Input: part model. Units: mm. Frame: model coordinates. A direction names the side the tool comes from. Coordinates: 2 decimals unless noted, no trailing zeros. Order: outer loops, then holes, each group sorted by start corner. A loop starts at its lowest first (then second) coordinate and runs counter-clockwise, first axis right, second up. Notation, with made-up numbers: (61, 58) -> (102, 58) arc R5 cw to (102, 64) -> close; hole circle Ø3 at (6, 7.25). An arc over 180 degrees is marked (long way). One line per question, with ' | ' between items.
```python
from build123d import *

# Parameters (mm, degrees)
BOSS_EXTRUDE18_DEPTH            = 24.1
CUT_EXTRUDE24_DEPTH             = 10.3
CUT_EXTRUDE25_DEPTH             = 8.9
BOSS_EXTRUDE7_DEPTH             = 9.3
CUT_EXTRUDE21_START             = -2
CUT_EXTRUDE21_DEPTH             = 2
BOSS_EXTRUDE2_REACH             = 48.304
SKETCH16_W                      = 40.7
SKETCH16_H                      = 7
BOSS_EXTRUDE2_DIRECTION_2_REACH = 48.304
BOSS_EXTRUDE3_REACH             = 58.743
SKETCH23_R                      = 3.5
BOSS_EXTRUDE3_DIRECTION_2_REACH = 58.743
SKETCH24_W                      = 12
SKETCH24_H                      = 5.4
SKETCH24_H_2                    = 3.45
CUT_EXTRUDE6_DEPTH              = 66.882774684
BOSS_EXTRUDE4_DEPTH             = 1
BOSS_EXTRUDE4_DEPTH_BACK        = 2.6
SKETCH28_R                      = 3
SKETCH33_W                      = 2.6
SKETCH33_H                      = 4
CUT_EXTRUDE10_DEPTH             = 5.4
CUT_EXTRUDE12_DEPTH             = 2.5
DELETEFACE7_START               = 23.1
DELETEFACE7_DEPTH               = 1
CUT_EXTRUDE29_START             = -1
SKETCH105_R                     = 1.7
CUT_EXTRUDE29_DEPTH             = 1
SKETCH106_W                     = 18
SKETCH106_H                     = 31.4
CUT_EXTRUDE30_DEPTH             = 2
CUT_EXTRUDE31_DEPTH             = 1.4


# Read off the part's stored shape, not the designer's step: DeleteFace7
with BuildPart() as part:
    # Sketch95 → Boss-Extrude18 (new body)
    with BuildSketch(Plane(origin=(0, 0, 0), x_dir=(0, 0, -1), z_dir=(1, 0, 0))):
        with BuildLine():
            Line((9, 29.5), (9, 7.1))
            Line((9, 7.1), (8.45, 7.1))
            Line((8.45, 7.1), (8.45, 0))
            Line((8.45, 0), (-8.45, 0))
            Line((-8.45, 0), (-8.45, 7.1))
            Line((-8.45, 7.1), (-9, 7.1))
            Line((-9, 7.1), (-9, 29.5))
            ThreePointArc((-9, 29.5), (0, 38.5), (9, 29.5))
        make_face()
    extrude(amount=BOSS_EXTRUDE18_DEPTH)

    # Sketch96 → Cut-Extrude24 (cut)
    with BuildSketch(Plane(origin=(24.1, 0, 0), x_dir=(0, 0, -1), z_dir=(1, 0, 0))):
        with BuildLine():
            Line((-7.45, 8.1), (-7.45, 1))
            Line((-7.45, 1), (7.45, 1))
            Line((7.45, 1), (7.45, 8.1))
            Line((7.45, 8.1), (8, 8.1))
            Line((8, 8.1), (8, 21.5))
            ThreePointArc((8, 21.5), (6.894427191, 23.288854382), (4.8, 23.1))
            ThreePointArc((4.8, 23.1), (0, 21.5), (-4.8, 23.1))
            ThreePointArc((-4.8, 23.1), (-6.894427191, 23.288854382), (-8, 21.5))
            Line((-8, 21.5), (-8, 8.1))
            Line((-8, 8.1), (-7.45, 8.1))
        make_face()
    extrude(amount=-CUT_EXTRUDE24_DEPTH, mode=Mode.SUBTRACT)

    # Sketch97 → Cut-Extrude25 (cut)
    with BuildSketch(Plane(origin=(24.1, 0, 0), x_dir=(0, 0, -1), z_dir=(1, 0, 0))):
        with BuildLine():
            Line((-8, 29.5), (-8, 21.5))
            Line((-8, 21.5), (8, 21.5))
            Line((8, 21.5), (8, 29.5))
            ThreePointArc((8, 29.5), (0, 37.5), (-8, 29.5))
        make_face()
    extrude(amount=-CUT_EXTRUDE25_DEPTH, mode=Mode.SUBTRACT)

    # Sketch11 → Cut-Revolve1 (revolve, cut)
    with BuildSketch(Plane.XY):
        Polygon((13.8, 14.5), (13.8, 9), (1.5, 9), (1.5, 10.25), (0, 10.25), (0, 14.5), align=None)
    revolve(axis=Axis((19.869277651, 14.5, 0), (-1, 0, 0)), mode=Mode.SUBTRACT)

    # Sketch12 → Cut-Revolve2 (revolve, cut)
    with BuildSketch(Plane.XY, mode=Mode.PRIVATE) as cut_revolve2_sk:
        Polygon((15.2, 29.5), (15.2, 26), (13.6, 26), (13.6, 22.25), (0, 22.25), (0, 29.5), align=None)
    revolve(cut_revolve2_sk.sketch.rotate(Axis((8.225974271, 29.5, 0), (1, 0, 0)), 270), axis=Axis((8.225974271, 29.5, 0), (1, 0, 0)), mode=Mode.SUBTRACT)

    # Sketch69 → Boss-Extrude7 (add)
    with BuildSketch(Plane(origin=(13.8, 0, 0), x_dir=(0, 0, -1), z_dir=(1, 0, 0))):
        with BuildLine():
            Line((8, 23.75), (8, 20.25))
            Line((8, 20.25), (6.25, 20.25))
            ThreePointArc((6.25, 20.25), (4.5, 22), (6.25, 23.75))
            Line((6.25, 23.75), (8, 23.75))
        make_face()
        with BuildLine():
            Line((-8, 23.75), (-8, 20.25))
            Line((-8, 20.25), (-6.25, 20.25))
            ThreePointArc((-6.25, 20.25), (-4.5, 22), (-6.25, 23.75))
            Line((-6.25, 23.75), (-8, 23.75))
        make_face()
        with BuildLine():
            Line((-4.6, 2.4), (-4.6, 1))
            Line((-4.6, 1), (-1.2, 1))
            Line((-1.2, 1), (-1.2, 2.4))
            ThreePointArc((-1.2, 2.4), (-2.9, 4.1), (-4.6, 2.4))
        make_face()
    extrude(amount=BOSS_EXTRUDE7_DEPTH)

    # Sketch80 → Cut-Extrude21 (cut)
    with BuildSketch(Plane(origin=(24.1, 0, 0), x_dir=(0, 0, -1), z_dir=(1, 0, 0)).offset(CUT_EXTRUDE21_START)):
        with BuildLine():
            Line((-7.45, 0), (-9, 0))
            Line((-9, 0), (-9, 8.1))
            Line((-9, 8.1), (-7.45, 8.1))
            Line((-7.45, 8.1), (-7.45, 2.4))
            Line((-7.45, 2.4), (-4.6, 2.4))
            ThreePointArc((-4.6, 2.4), (-2.9, 0.7), (-1.2, 2.4))
            Line((-1.2, 2.4), (7.45, 2.4))
            Line((7.45, 2.4), (7.45, 8.1))
            Line((7.45, 8.1), (9, 8.1))
            Line((9, 8.1), (9, 0))
            Line((9, 0), (7.45, 0))
            Line((7.45, 0), (-7.45, 0))
        make_face()
    extrude(amount=CUT_EXTRUDE21_DEPTH, mode=Mode.SUBTRACT)

    # Boss-Extrude2: up to this face of the body (flat: up to its plane)
    boss_extrude2_end = Plane(part.part.faces().sort_by_distance((11.05, 3.55, 8.45))[0])
    # Sketch16 → Boss-Extrude2 (add, up to the picked face)
    with BuildSketch(Plane.XY, mode=Mode.PRIVATE) as boss_extrude2_sk1:
        with Locations((-20.35, 3.5)):
            Rectangle(SKETCH16_W, SKETCH16_H)
    boss_extrude2_tool1 = split(extrude(boss_extrude2_sk1.sketch, amount=BOSS_EXTRUDE2_REACH, mode=Mode.PRIVATE), bisect_by=boss_extrude2_end, keep=Keep.BOTH, mode=Mode.PRIVATE)
    add(boss_extrude2_tool1.solids().sort_by(Axis((-20.35, 3.5, 0), (0, 0, 1)))[0])

    # Boss-Extrude2 direction 2: up to this face of the body (flat: up to its plane)
    boss_extrude2_direction_2_end = Plane(part.part.faces().sort_by_distance((11.05, 3.55, -8.45))[0])
    # Sketch16 → Boss-Extrude2 direction 2 (add, up to the picked face)
    with BuildSketch(Plane.XY, mode=Mode.PRIVATE) as boss_extrude2_direction_2_sk1:
        with Locations((-20.35, 3.5)):
            Rectangle(SKETCH16_W, SKETCH16_H)
    boss_extrude2_direction_2_tool1 = split(extrude(boss_extrude2_direction_2_sk1.sketch, amount=-BOSS_EXTRUDE2_DIRECTION_2_REACH, mode=Mode.PRIVATE), bisect_by=boss_extrude2_direction_2_end, keep=Keep.BOTH, mode=Mode.PRIVATE)
    add(boss_extrude2_direction_2_tool1.solids().sort_by(Axis((-20.35, 3.5, 0), (0, 0, -1)))[0])

    # Boss-Extrude3: up to this face of the body (flat: up to its plane)
    boss_extrude3_end = Plane(part.part.faces().sort_by_distance((-9.198206243, 3.517757633, 8.45))[0])
    # Sketch23 → Boss-Extrude3 (add, up to the picked face)
    with BuildSketch(Plane.XY, mode=Mode.PRIVATE) as boss_extrude3_sk1:
        with BuildLine():
            Line((-41.908497378, 7), (-40.7, 7))
            Line((-40.7, 7), (-40.7, 0))
            Line((-40.7, 0), (-47.2, 0))
            ThreePointArc((-47.2, 0), (-51.587482194, 8.81662479), (-41.908497378, 7))
        make_face()
        with Locations(Location((-47.2, 5.5, 0), (0, 0, 180))):
            Circle(SKETCH23_R, mode=Mode.SUBTRACT)
    boss_extrude3_tool1 = split(extrude(boss_extrude3_sk1.sketch, amount=BOSS_EXTRUDE3_REACH, mode=Mode.PRIVATE), bisect_by=boss_extrude3_end, keep=Keep.BOTH, mode=Mode.PRIVATE)
    add(boss_extrude3_tool1.solids().sort_by(Axis((-41.304249, 6.837212, 0), (0, 0, 1)))[0])

    # Boss-Extrude3 direction 2: up to this face of the body (flat: up to its plane)
    boss_extrude3_direction_2_end = Plane(part.part.faces().sort_by_distance((-9.198206243, 3.517757633, -8.45))[0])
    # Sketch23 → Boss-Extrude3 direction 2 (add, up to the picked face)
    with BuildSketch(Plane.XY, mode=Mode.PRIVATE) as boss_extrude3_direction_2_sk1:
        with BuildLine():
            Line((-41.908497378, 7), (-40.7, 7))
            Line((-40.7, 7), (-40.7, 0))
            Line((-40.7, 0), (-47.2, 0))
            ThreePointArc((-47.2, 0), (-51.587482194, 8.81662479), (-41.908497378, 7))
        make_face()
        with Locations(Location((-47.2, 5.5, 0), (0, 0, 180))):
            Circle(SKETCH23_R, mode=Mode.SUBTRACT)
    boss_extrude3_direction_2_tool1 = split(extrude(boss_extrude3_direction_2_sk1.sketch, amount=-BOSS_EXTRUDE3_DIRECTION_2_REACH, mode=Mode.PRIVATE), bisect_by=boss_extrude3_direction_2_end, keep=Keep.BOTH, mode=Mode.PRIVATE)
    add(boss_extrude3_direction_2_tool1.solids().sort_by(Axis((-41.304249, 6.837212, 0), (0, 0, -1)))[0])

    # Sketch24 → Cut-Extrude6 (cut, through all)
    with BuildSketch(Plane(origin=(0, 0, 0), x_dir=(1, 0, 0), z_dir=(0, 1, 0))):
        with Locations((-46.7, 0)):
            Rectangle(SKETCH24_W, SKETCH24_H)
        with Locations((-46.7, -6.725)):
            Rectangle(SKETCH24_W, SKETCH24_H_2)
        with Locations((-46.7, 6.725)):
            Rectangle(SKETCH24_W, SKETCH24_H_2)
    extrude(amount=CUT_EXTRUDE6_DEPTH, mode=Mode.SUBTRACT)

    # Sketch28 → Boss-Extrude4 (add, two sides: drawn at the far end of the back side and taken through both)
    with BuildSketch(Plane(origin=(-40.7, 0, 0), x_dir=(0, 0, -1), z_dir=(1, 0, 0)).offset(-BOSS_EXTRUDE4_DEPTH_BACK)):
        with BuildLine():
            Line((-5, 7), (5, 7))
            Line((5, 7), (5, 14.5))
            ThreePointArc((5, 14.5), (0, 19.5), (-5, 14.5))
            Line((-5, 14.5), (-5, 7))
        make_face()
        with Locations((0, 14.5)):
            Circle(SKETCH28_R, mode=Mode.SUBTRACT)
    extrude(amount=BOSS_EXTRUDE4_DEPTH + BOSS_EXTRUDE4_DEPTH_BACK)

    # Sketch33 → Cut-Extrude10 (cut)
    with BuildSketch(Plane.XY.offset(-2.7)):
        with Locations((-42, 7)):
            Rectangle(SKETCH33_W, SKETCH33_H)
    extrude(amount=CUT_EXTRUDE10_DEPTH, mode=Mode.SUBTRACT)

    # Sketch35 → Cut-Extrude12 (cut)
    with BuildSketch(Plane(origin=(0, 7, 0), x_dir=(1, 0, 0), z_dir=(0, 1, 0))):
        Polygon((-36.6, 2.65), (-38.1, 2.65), (-38.1, -2.65), (-36.6, -2.65), (-8.3, -2.65), (-6.8, -2.65), (-6.8, 2.65), (-8.3, 2.65), align=None)
    extrude(amount=-CUT_EXTRUDE12_DEPTH, mode=Mode.SUBTRACT)

    # DeleteFace7 outline → DeleteFace7 (cut)
    with BuildSketch(Plane.YZ.offset(DELETEFACE7_START)):
        with BuildLine():
            Line((1, 1.935634924), (1, 3.864365076))
            ThreePointArc((1, 3.864365076), (0.7, 2.9), (1, 1.935634924))
        make_face()
    extrude(amount=DELETEFACE7_DEPTH, mode=Mode.SUBTRACT)

    # Sketch105 → Cut-Extrude29 (cut)
    with BuildSketch(Plane(origin=(23.1, 0, 0), x_dir=(0, 0, -1), z_dir=(1, 0, 0)).offset(CUT_EXTRUDE29_START)):
        with Locations((-2.9, 2.4)):
            Circle(SKETCH105_R)
    extrude(amount=CUT_EXTRUDE29_DEPTH, mode=Mode.SUBTRACT)

    # Sketch106 → Cut-Extrude30 (cut)
    with BuildSketch(Plane(origin=(24.1, 0, 0), x_dir=(0, 0, -1), z_dir=(1, 0, 0))):
        with Locations((0, 22.8)):
            Rectangle(SKETCH106_W, SKETCH106_H)
    extrude(amount=-CUT_EXTRUDE30_DEPTH, mode=Mode.SUBTRACT)

    # Sketch107 → Cut-Extrude31 (cut)
    with BuildSketch(Plane(origin=(15.2, 0, 0), x_dir=(0, 0, -1), z_dir=(1, 0, 0))):
        with BuildLine():
            Line((-6.25, 23.75), (6.25, 23.75))
            ThreePointArc((6.25, 23.75), (5.583042256, 23.617920693), (5.016760303, 23.241619849))
            ThreePointArc((5.016760303, 23.241619849), (4.906085954, 23.174321373), (4.8, 23.1))
            ThreePointArc((4.8, 23.1), (0, 21.5), (-4.8, 23.1))
            ThreePointArc((-4.8, 23.1), (-4.906085954, 23.174321373), (-5.016760303, 23.241619849))
            ThreePointArc((-5.016760303, 23.241619849), (-5.583042256, 23.617920693), (-6.25, 23.75))
        make_face()
    extrude(amount=-CUT_EXTRUDE31_DEPTH, mode=Mode.SUBTRACT)


solid = part.part
```
1. Mould query, pull axis Z, two halves, no side actions, for faces 4 (the face through (18, 14, 8)), 5 (the face through (-50.433, 6.841, -3.834)), 6 (the face through (-10, 4, 8.45)). Classes: released by +Z, released by -Z, zero draft, split by the parting line, or undercut.
Recorded:
face 4: undercut | face 5: zero draft | face 6: released by +Z
2. Cut plane D-D, the plane x = -2.5. Return loops of the section in (y, z).
Recorded:
outline: (0, -8.45) -> (7, -8.45) -> (7, 8.45) -> (0, 8.45) -> close
3. Cut plane C-C, the plane z = -1.5. State how many separate pieces and enclosed holes the cut face has, and give its area (3 significant figures).
Recorded:
separate pieces: 4 | enclosed holes: 0 | area: 447 mm^2
4. Ray query, line 1 (X direction, y = 5.5, z = -3.6); line 2 (Z direction, x = 18.5, y = 2.5); line 3 (Z direction, x = 9.75, y = 14.5). Return the intervals inside material, ascending. Write a range as [from, to].
Recorded:
line 1: x = [-52.7, -50.7], [-43.7, 13.8] | line 2: z = [-8.45, -7.45], [1.2, 4.6], [7.45, 8.45] | line 3: z = [-9, -5.5], [5.5, 9]
5. Access query for faces 1 (the face through (18, 1, 6)), 2 (the face through (-6.8, 6, 0)), 3 (the face through (-39.7, 11, 0)). Directions: +Z, -Z, +X, -X, +Y, -Y. A direction counts if a zero-diameter tool reaches every point of the face in a straight line with its end or side. Return the directions, or none.
Recorded:
face 1: +X | face 2: +Y | face 3: +Z, -Z, +Y
6. Pin query (flat end, axial travel): pin 1 Ø8 at (y, z) = (33, -5) entering from -X; pin 2 Ø3 at (y, z) = (27.5, 1) entering from -X; pin 3 Ø3.5 at (y, z) = (14.5, 0) entering from +X; pin 4 Ø2.5 at (x, z) = (17.5, 6) entering from +Y. Return the tip coordinate at first contact, or that it passes through.
Recorded:
pin 1: stops at x = 0 | pin 2: stops at x = 13.6 | pin 3: passes through | pin 4: stops at y = 37.14
7. Cut plane B-B, the plane x = -22. Return loops of the section in (y, z), and give its area (3 significant figures).
Recorded:
outline: (0, -8.45) -> (7, -8.45) -> (7, -2.65) -> (4.5, -2.65) -> (4.5, 2.65) -> (7, 2.65) -> (7, 8.45) -> (0, 8.45) -> close | area: 105 mm^2
8. Cut plane A-A, the plane x = 16. Return loops of the section in (y, z).
Recorded:
outline: (0, -8.45) -> (7.1, -8.45) -> (7.1, -9) -> (29.5, -9) arc R9 ccw to (29.5, 9) -> (7.1, 9) -> (7.1, 8.45) -> (0, 8.45) -> close; hole (1, -7.45) -> (8.1, -7.45) -> (8.1, -8) -> (20.25, -8) -> (20.25, -6.25) arc R1.75 cw to (23.75, -6.25) -> (23.75, -8) -> (29.5, -8) arc R8 ccw to (29.5, 8) -> (23.75, 8) -> (23.75, 6.25) arc R1.75 cw to (20.25, 6.25) -> (20.25, 8) -> (8.1, 8) -> (8.1, 7.45) -> (1, 7.45) -> (1, 4.6) -> (2.4, 4.6) arc R1.7 cw to (2.4, 1.2) -> (1, 1.2) -> close
